CAD build for the part. Positions are in the model's coordinates, mm. Face numbers are marked on the shaded views. A direction names the side the tool comes from. Give positions to 0.01 mm unless a question says otherwise; leave off trailing zeros. Loops run counter-clockwise (first coordinate to the right, second up) from the corner with the lowest first, then second, coordinate; pieces in that order, holes last. Notation, with made-up numbers: (44, 15.25) -> (95, 15.25) arc R4 cw to (95, 20.25) -> close; hole circle Ø4 at (-17, 14). An arc over 180 degrees is marked (long way). Use one line per item in the form item = value.
```python
from build123d import *

# Parameters (mm, degrees)
SKETCH1_W           = 18
SKETCH1_H           = 21
SKETCH1_R           = 2.1
BOSS_EXTRUDE1_DEPTH = 4
CUT_EXTRUDE1_DEPTH  = 4
CHAMFER1_SIZE       = 1.75
FILLET1_R           = 2
CHAMFER2_SIZE       = 3
CHAMFER3_SIZE       = 1
FILLET2_R           = 2


with BuildPart() as part:
    # Sketch1 → Boss-Extrude1 (new body)
    with BuildSketch(Plane(origin=(0, 0, 0), x_dir=(0, 0, -1), z_dir=(1, 0, 0))):
        Rectangle(SKETCH1_W, SKETCH1_H)
        with Locations((5.5, 4.5)):
            Circle(SKETCH1_R, mode=Mode.SUBTRACT)
        with Locations((-5.5, 4.846153846)):
            Circle(SKETCH1_R, mode=Mode.SUBTRACT)
    extrude(amount=BOSS_EXTRUDE1_DEPTH)

    # Sketch2 → Cut-Extrude1 (cut)
    with BuildSketch(Plane(origin=(4, 0, 0), x_dir=(0, 0, -1), z_dir=(1, 0, 0))):
        with BuildLine():
            Line((6.8, -1.316455335), (6.8, -7.014826284))
            ThreePointArc((6.8, -7.014826284), (5, -8.814826284), (3.2, -7.014826284))
            Line((3.2, -7.014826284), (3.2, -1.316455335))
            ThreePointArc((3.2, -1.316455335), (5, 0.483544665), (6.8, -1.316455335))
        make_face()
        with BuildLine():
            Line((-3.2, -1.316455335), (-3.2, -7.014826284))
            ThreePointArc((-3.2, -7.014826284), (-5, -8.814826284), (-6.8, -7.014826284))
            Line((-6.8, -7.014826284), (-6.8, -1.316455335))
            ThreePointArc((-6.8, -1.316455335), (-5, 0.483544665), (-3.2, -1.316455335))
        make_face()
    extrude(amount=-CUT_EXTRUDE1_DEPTH, mode=Mode.SUBTRACT)

    # Chamfer1
    # the kernel refuses this chamfer: 1.75 mm, written as the material it takes off along each edge
    with BuildSketch(Plane(origin=(4, -1.316455335, -5), x_dir=(0, 0, 1), z_dir=(0, -1, 0))) as chamfer1_piece_1:
        Polygon((1.8 + CHAMFER1_SIZE, 0), (1.8, CHAMFER1_SIZE), (1.8, 0), align=None)
    revolve(axis=Axis((4, -1.316455335, -5), (-1, 0, 0)), revolution_arc=180, mode=Mode.SUBTRACT)
    with BuildSketch(Plane(origin=(4, -7.014826284, -3.2), x_dir=(0.02749587661058661, 0, 0.9996219169112968), z_dir=(0, 1, 0)), Plane(origin=(4, -1.316455335, -6.8), x_dir=(0.027495876610586112, 0, -0.9996219169112968), z_dir=(0, -1, 0)), Plane(origin=(4, -7.014826284, 6.8), x_dir=(0.02749587661058662, 0, 0.9996219169112968), z_dir=(0, 1, 0)), Plane(origin=(4, -1.316455335, 3.2), x_dir=(0.02749587661058661, 0, -0.9996219169112968), z_dir=(0, -1, 0))) as chamfer1_piece_2:
        Polygon((CHAMFER1_SIZE * 0.999621916911, -CHAMFER1_SIZE * 0.0274958766106), (-CHAMFER1_SIZE * 0.0274958766106, -CHAMFER1_SIZE * 0.999621916911), (0, 0), align=None)
    extrude(amount=5.698370949, mode=Mode.SUBTRACT)
    with BuildSketch(Plane(origin=(4, -7.014826284, -5), x_dir=(0, 0, -1), z_dir=(0, 1, 0))) as chamfer1_piece_3:
        Polygon((1.8 + CHAMFER1_SIZE, 0), (1.8, CHAMFER1_SIZE), (1.8, 0), align=None)
    revolve(axis=Axis((4, -7.014826284, -5), (-1, 0, 0)), revolution_arc=180, mode=Mode.SUBTRACT)
    with BuildSketch(Plane(origin=(4, -1.316455335, 5), x_dir=(0, 0, 1), z_dir=(0, -1, 0))) as chamfer1_piece_4:
        Polygon((1.8 + CHAMFER1_SIZE, 0), (1.8, CHAMFER1_SIZE), (1.8, 0), align=None)
    revolve(axis=Axis((4, -1.316455335, 5), (-1, 0, 0)), revolution_arc=180, mode=Mode.SUBTRACT)
    with BuildSketch(Plane(origin=(4, -7.014826284, 5), x_dir=(0, 0, -1), z_dir=(0, 1, 0))) as chamfer1_piece_5:
        Polygon((1.8 + CHAMFER1_SIZE, 0), (1.8, CHAMFER1_SIZE), (1.8, 0), align=None)
    revolve(axis=Axis((4, -7.014826284, 5), (-1, 0, 0)), revolution_arc=180, mode=Mode.SUBTRACT)

    # Fillet1
    fillet1_edges = [part.edges().sort_by_distance(p)[0] for p in [
        (2, -10.5, -9),
        (2, -10.5, 9),
        (2, 10.5, 9),
        (2, 10.5, -9),
    ]]
    fillet(fillet1_edges, radius=FILLET1_R)

    # Chamfer2
    # the kernel refuses this chamfer: 3 mm, written as the material it takes off along each edge
    with BuildSketch(Plane(origin=(0, 10.5, 14.715048964), x_dir=(0.9996219169112968, 0.027495876610586202, 0), z_dir=(0, 0, -1))) as chamfer2_piece_1:
        Polygon((CHAMFER2_SIZE * 0.999621916911, CHAMFER2_SIZE * 0.0274958766106), (-CHAMFER2_SIZE * 0.0274958766106, CHAMFER2_SIZE * 0.999621916911), (0, 0), align=None)
    extrude(amount=29.430097928, mode=Mode.SUBTRACT)

    # Chamfer3
    chamfer3_edges = [part.edges().sort_by_distance(p)[0] for p in [
        (0, -0.5, -9),
        (0, -9.914213562, -8.414213562),
        (0, -10.5, 0),
        (0, -9.914213562, 8.414213562),
        (0, -0.5, 9),
    ]]
    chamfer(chamfer3_edges, length=CHAMFER3_SIZE)

    # Fillet2
    fillet2_edges = [part.edges().sort_by_distance(p)[0] for p in [
        (0.5, 8, -8.5),
        (0.5, 8, 8.5),
    ]]
    fillet(fillet2_edges, radius=FILLET2_R)


solid = part.part
```
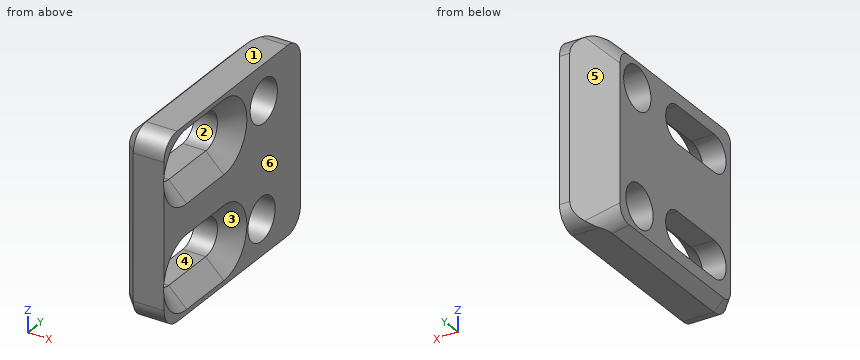
1. Drill centre lines: line 1 (Z direction, x = 3.7, y = 5); line 2 (Y direction, x = 2.1, z = -4.25); line 3 (Z direction, x = 2.9, y = 0.5). Where is each one in solid material? Low to high.
Result sheet:
line_1 = -9 to -7.54, -3.46 to 3.41, 7.59 to 9
line_2 = -10.5 to -8.65, 0.32 to 2.81, 6.19 to 9.6
line_3 = -9 to -6.64, -3.36 to 3.36, 6.64 to 9
2. Cut at C-C, the plane z = 5. Write the cut outline in (x, y).
Result sheet:
outline = (0, -9.5) -> (1, -10.5) -> (3.94, -10.5) -> (2.25, -8.81) -> (0, -8.81) -> close; (0, 0.48) -> (2.25, 0.48) -> (4, 2.23) -> (4, 2.81) -> (0, 2.81) -> close; (0, 6.89) -> (4, 6.89) -> (4, 10.5) -> (3, 10.5) -> (0, 7.5) -> close
3. Mould opens along Y. For the marked faces 4, 5 and 6 say: pulls with the +Y half, pulls with the -Y half, needs draft (parallel to the pull), parting line crosses it, or undercut.
Result sheet:
face_4 = undercut
face_5 = pulls with the +Y half
face_6 = needs draft
4. Cut at D-D, the plane y = 5.75. Write the cut outline in (x, z).
Result sheet:
outline = (0, -8) -> (1, -9) -> (4, -9) -> (4, -7.19) -> (0, -7.19) -> close; (0, -3.81) -> (4, -3.81) -> (4, 3.6) -> (0, 3.6) -> close; (0, 7.4) -> (4, 7.4) -> (4, 9) -> (1, 9) -> (0, 8) -> close
5. Cut at B-B, the plane x = 3.5. Write the cut outline in (y, z).
Result sheet:
outline = (-10.5, -7) arc R2 ccw to (-8.5, -9) -> (8.5, -9) arc R2 ccw to (10.5, -7) -> (10.5, 7) arc R2 ccw to (8.5, 9) -> (-8.5, 9) arc R2 ccw to (-10.5, 7) -> close; hole (-7.01, -8.05) -> (-1.32, -8.05) arc R3.05 ccw to (-1.32, -1.95) -> (-7.01, -1.95) arc R3.05 ccw to start; hole (-7.01, 1.95) -> (-1.32, 1.95) arc R3.05 ccw to (-1.32, 8.05) -> (-7.01, 8.05) arc R3.05 ccw to start; hole circle Ø4.2 at (4.5, -5.5); hole circle Ø4.2 at (4.85, 5.5)
6. Cut at A-A, the plane y = -5.25. Write the cut outline in (x, z).
Result sheet:
outline = (0, -8) -> (1, -9) -> (4, -9) -> (4, -8.55) -> (2.25, -6.8) -> (0, -6.8) -> close; (0, -3.2) -> (2.25, -3.2) -> (4, -1.45) -> (4, 1.45) -> (2.25, 3.2) -> (0, 3.2) -> close; (0, 6.8) -> (2.25, 6.8) -> (4, 8.55) -> (4, 9) -> (1, 9) -> (0, 8) -> close
7. Tool access for the marked faces 1, 2 and 3: list every direction of +Z, -Z, +X, -X, +Y, -Y with a clear straight run to the whole face (end or side of a thin tool).
Result sheet:
face_1 = +Z, +X, -X, +Y, -Y
face_2 = +X, -X
face_3 = +X
